Check sheet for the modelled part. Datum: model origin and axes. Units: mm. Face numbers are marked on the shaded views. A direction names the side the tool comes from. Round coordinates to 2 decimals unless told otherwise and drop trailing zeros. Order: outer loops, then holes, each group sorted by start corner. A loop starts at its lowest first (then second) coordinate and runs counter-clockwise, first axis right, second up.
(1) Sectioned sample at B-B, the plane x = 6.5. Enter the section's corners in (y, z), and give its area (4 significant figures).
(2) Thickness scan on probe 1 along X at (y, z) = (23.25, 0); probe 2 along X at (y, z) = (1.75, 14); probe 3 along Z at (x, y) = (15, 1.15). Record the ranges inside material, lowest first.
(3) Mould release check, pull along X, two halves, no side actions. Record for the marked faces 1, 2 and 3: released by +X, released by -X, zero draft, split by the parting line, or undercut.
(4) Sectioned sample at A-A, the plane z = 0. Enter the section's corners in (x, y), and give its area (3 significant figures).
(5) Depth check by flat-ended pin: pin 1 (6 mm diameter, centred on x = -18.5, y = 16, fed in from -Z); pin 2 (3 mm diameter, centred on x = -19, y = 17.5, fed in from -Z); pin 3 (2 mm diameter, centred on x = -15, z = -15, fed in from +Y). Enter the tip coordinate at first touch or a pass-through.
(6) Tool access check on the marked faces 4, 5 and 6. Record the directions out of +Z, -Z, +X, -X, +Y, -Y that give a thin tool (end or side, any length) a straight path to the whole face; none if there is none.
```python
from build123d import *

# Parameters (mm, degrees)
SKETCH1_R                 = 17
BOSS_EXTRUDE1_DEPTH       = 21
SKETCH2_R                 = 20
BOSS_EXTRUDE2_DEPTH       = 8
CUT_EXTRUDE3_DEPTH        = 8
M3_TAPPED_HOLE1_D         = 2.5
M3_TAPPED_HOLE1_DEPTH     = 10
M3_TAPPED_HOLE1_TIP       = 0.751075774
F_4_40_TAPPED_HOLE1_D     = 2.2606
F_4_40_TAPPED_HOLE1_DEPTH = 5
F_4_40_TAPPED_HOLE1_TIP   = 0.679152758
M3X0_2_TAPPED_HOLE1_D     = 2.8
M3X0_2_TAPPED_HOLE2_D     = 2.8
CUT_EXTRUDE4_REACH        = 52
SKETCH20_R                = 2
CUT_EXTRUDE5_DEPTH        = 12


with BuildPart() as part:
    # Sketch1 → Boss-Extrude1 (new body)
    with BuildSketch(Plane(origin=(0, 0, 0), x_dir=(1, 0, 0), z_dir=(0, 1, 0))):
        Polygon((10.355339059, 25), (-10.355339059, 25), (-25, 10.355339059), (-25, -10.355339059), (-10.355339059, -25), (10.355339059, -25), (25, -10.355339059), (25, 10.355339059), align=None)
        Circle(SKETCH1_R, mode=Mode.SUBTRACT)
    extrude(amount=BOSS_EXTRUDE1_DEPTH)

    # Sketch2 → Boss-Extrude2 (add)
    with BuildSketch(Plane(origin=(0, 21, 0), x_dir=(1, 0, 0), z_dir=(0, 1, 0))):
        Polygon((25, 10.355339059), (10.355339059, 25), (-10.355339059, 25), (-25, 10.355339059), (-25, -10.355339059), (-10.355339059, -25), (10.355339059, -25), (25, -10.355339059), align=None)
        Circle(SKETCH2_R, mode=Mode.SUBTRACT)
    extrude(amount=BOSS_EXTRUDE2_DEPTH)

    # Sketch6 → Cut-Extrude3 (cut)
    with BuildSketch(Plane(origin=(0, 29, 0), x_dir=(1, 0, 0), z_dir=(0, 1, 0))):
        Polygon((-19.940411229, 15.41492783), (-16.222684393, 11.697200993), (16.222684393, 11.697200993), (19.940411229, 15.41492783), (10.355339059, 25), (-10.355339059, 25), align=None)
    extrude(amount=-CUT_EXTRUDE3_DEPTH, mode=Mode.SUBTRACT)

    # M3 Tapped Hole1
    with Locations(Plane(origin=(0, 29, 0), x_dir=(1, 0, 0), z_dir=(0, 1, 0))):
        with Locations((20.842542104, 8.633263614), (-20.842542104, 8.633263614), (-8.633263614, -20.842542104), (8.633263614, -20.842542104)):
            Hole(M3_TAPPED_HOLE1_D / 2, depth=M3_TAPPED_HOLE1_DEPTH)
            with Locations((0, 0, -(M3_TAPPED_HOLE1_DEPTH + M3_TAPPED_HOLE1_TIP / 2))):  # 118° drill point
                Cone(0, M3_TAPPED_HOLE1_D / 2, M3_TAPPED_HOLE1_TIP, mode=Mode.SUBTRACT)

    # #4-40 Tapped Hole1
    with Locations(Plane(origin=(0, 0, 0), x_dir=(-1, 0, 0), z_dir=(0, -1, 0))):
        with Locations((-15, 15), (15, 15), (-15, -15), (15, -15)):
            Hole(F_4_40_TAPPED_HOLE1_D / 2, depth=F_4_40_TAPPED_HOLE1_DEPTH)
            with Locations((0, 0, -(F_4_40_TAPPED_HOLE1_DEPTH + F_4_40_TAPPED_HOLE1_TIP / 2))):  # 118° drill point
                Cone(0, F_4_40_TAPPED_HOLE1_D / 2, F_4_40_TAPPED_HOLE1_TIP, mode=Mode.SUBTRACT)

    # M3x0.2 Tapped Hole1 (through all)
    with Locations(Plane(origin=(17.67766953, 0, -17.67766953), x_dir=(-0.707106781, 0, -0.707106781), z_dir=(0.707106781, 0, -0.707106781))):
        with Locations((0, 11)):
            Hole(M3X0_2_TAPPED_HOLE1_D / 2)

    # M3x0.2 Tapped Hole2 (through all)
    with Locations(Plane(origin=(-17.67766953, 0, -17.67766953), x_dir=(-0.707106781, 0, 0.707106781), z_dir=(-0.707106781, 0, -0.707106781))):
        with Locations((0, 13.5)):
            Hole(M3X0_2_TAPPED_HOLE2_D / 2)

    # Sketch20 → Cut-Extrude4 (cut, up to next)
    with BuildSketch(Plane.XY.offset(25), mode=Mode.PRIVATE) as cut_extrude4_sk1:
        with Locations((0, 10)):
            Circle(SKETCH20_R)
    cut_extrude4_tool1 = extrude(cut_extrude4_sk1.sketch, amount=-CUT_EXTRUDE4_REACH, mode=Mode.PRIVATE) & part.part
    add(cut_extrude4_tool1.solids().sort_by_distance((0, 10, 25))[0], mode=Mode.SUBTRACT)

    # Sketch22 → Cut-Extrude5 (cut)
    with BuildSketch(Plane(origin=(0, 29, 0), x_dir=(1, 0, 0), z_dir=(0, 1, 0))):
        with BuildLine():
            Line((-17.67766953, 17.67766953), (-17.67766953, 26.402318696))
            Line((-17.67766953, 26.402318696), (17.67766953, 26.402318696))
            Line((17.67766953, 26.402318696), (17.67766953, 17.67766953))
            ThreePointArc((17.67766953, 17.67766953), (0, 25), (-17.67766953, 17.67766953))
        make_face()
    extrude(amount=-CUT_EXTRUDE5_DEPTH, mode=Mode.SUBTRACT)


solid = part.part
```
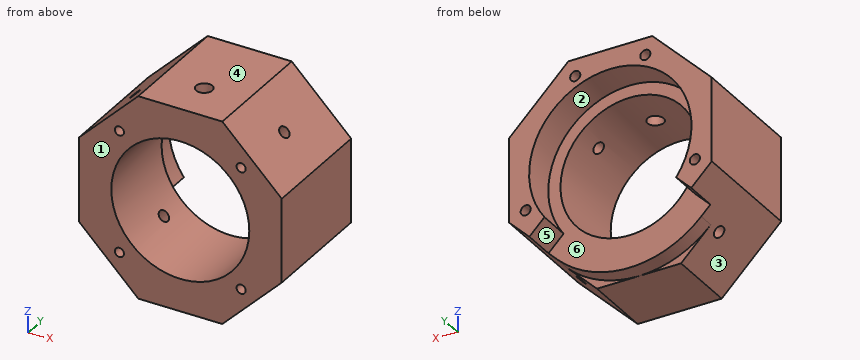
Derived:
1. outline: (0, -25) - (17, -25) - (17, -24.14) - (21, -24.14) - (21, -15.71) - (0, -15.71) - close; (0, 15.71) - (21, 15.71) - (21, 18.91) - (29, 18.91) - (29, 25) - (0, 25) - close
1. area: 435.5 mm2
2. probe 1: x = -25 to -20, 20 to 25
2. probe 2: x = -21.36 to -15.53, -14.47 to -9.64, 9.64 to 14.47, 15.53 to 21.36
2. probe 3: z = -20.36 to -16.13, -13.87 to -8, 8 to 13.87, 16.13 to 20.36
3. face 1: zero draft
3. face 2: undercut
3. face 3: released by -X
4. outline: (-25, 0) - (-17, 0) - (-17, 21) - (-20, 21) - (-20, 29) - (-25, 29) - close; (17, 0) - (25, 0) - (25, 29) - (20, 29) - (20, 21) - (17, 21) - close
4. area: 416 mm2
5. pin 1: stops at z = -19.86
5. pin 2: stops at z = -17.85
5. pin 3: stops at y = 21
6. face 4: +Z, +X, -X, +Y, -Y
6. face 5: -Z, +Y
6. face 6: +Y
